```python
from build123d import *

# Parameters (mm, degrees)
SKETCH1_W           = 254
SKETCH1_H           = 31.75
SKETCH1_R           = 3.048
BOSS_EXTRUDE1_DEPTH = 2.54
CHAMFER1_SIZE       = 2.38
CHAMFER1_SIZE_2     = 4.122280922
SKETCH3_W           = 254
SKETCH3_H           = 12.7
BOSS_EXTRUDE2_DEPTH = 1.016
BOSS_EXTRUDE3_DEPTH = 1.016


with BuildPart() as part:
    # Sketch1 → Boss-Extrude1 (new body)
    with BuildSketch(Plane.XY):
        with Locations((127, 22.225)):
            Rectangle(SKETCH1_W, SKETCH1_H)
        with Locations((121.412, 12.7)):
            Circle(SKETCH1_R, mode=Mode.SUBTRACT)
        with Locations((248.412, 12.7)):
            Circle(SKETCH1_R, mode=Mode.SUBTRACT)
    extrude(amount=BOSS_EXTRUDE1_DEPTH)

    # Chamfer1
    # the kernel refuses this chamfer: 4.122280922, 2.38 mm, written as the material it takes off along each edge
    with BuildSketch(Plane(origin=(264.66469425, 6.35, 2.54), x_dir=(0, -0.05789386240267149, -0.9983227437537926), z_dir=(-1, 0, 0))) as chamfer1_piece_1:
        Polygon((CHAMFER1_SIZE * 0.998322743754, -CHAMFER1_SIZE * 0.0578938624027), (-CHAMFER1_SIZE_2 * 0.0578938624029, -CHAMFER1_SIZE_2 * 0.998322743757), (0, 0), align=None)
    extrude(amount=275.3293885, mode=Mode.SUBTRACT)

    # Sketch3 → Boss-Extrude2 (add)
    with BuildSketch(Plane(origin=(0, 0, 0), x_dir=(-1, 0, 0), z_dir=(0, 0, -1))):
        with Locations((-127, 31.75)):
            Rectangle(SKETCH3_W, SKETCH3_H)
    extrude(amount=BOSS_EXTRUDE2_DEPTH)

    # Sketch4 → Boss-Extrude3 (add)
    with BuildSketch(Plane(origin=(0, 0, 0), x_dir=(-1, 0, 0), z_dir=(0, 0, -1))):
        Polygon((0, 25.4), (0, 6.35), (-3.556, 6.35), (-14.224, 25.4), align=None)
    extrude(amount=BOSS_EXTRUDE3_DEPTH)


solid = part.part
```
The listing builds one solid part. Answer for the finished solid, in the listing's coordinates (mm). A direction names the side the tool comes from. Give positions to 0.01 mm unless a question says otherwise; leave off trailing zeros. Loops run counter-clockwise (first coordinate to the right, second up) from the corner with the lowest first, then second, coordinate; pieces in that order, holes last. Notation, with made-up numbers: M 82.25,26.5 L 137.25,26.5 A12 cw 137.25,49.5 Z; hole C -36,-39.75 d11. An arc over 180 degrees is marked long. One line per item, written item: value.
Q1. For faces 4 (the face through (125, 30, -1.016)), 5 (the face through (127, 16, 0)), determine the directions among +Z, -Z, +X, -X, +Y, -Y from which every point of the face is accessible in a straight line to the end or side of a thin tool.
Working result:
face 4: -Z, +X, -X, +Y, -Y
face 5: -Z, +X, -Y
Q2. A cutting plane is placed at A-A on x = 87. Determine the outline of the cut face in (y, z), then the cut area to 3 significant figures.
Working result:
outline: M 6.35,0 L 25.4,0 L 25.4,-1.02 L 38.1,-1.02 L 38.1,2.54 L 10.47,2.54 L 6.35,0.16 Z
area: 88.6 mm^2
Q3. A cutting plane is placed at B-B on y = 12.7. Determine the outline of the cut face in (x, z).
Working result:
outline: M 0,-1.02 L 7.11,-1.02 L 7.11,0 L 118.36,0 L 118.36,2.54 L 0,2.54 Z; M 124.46,0 L 245.36,0 L 245.36,2.54 L 124.46,2.54 Z; M 251.46,0 L 254,0 L 254,2.54 L 251.46,2.54 Z
Q4. Determine the mould class of faces 1 (the face through (121.015, 15.722, 1.252)), 2 (the face through (8.815, 15.742, -0.501)), 3 (the face through (125, 24, 2.54)) for opening direction X: +X half, -X half, draft (parallel to the pull), parting line (faces both ways), or undercut.
Working result:
face 1: undercut
face 2: +X half
face 3: draft
Q5. Find the intervals of material crossed by line 1 (X direction, y = 12.7, z = 1.8); line 2 (Y direction, x = 217.5, z = -0.4); line 3 (Z direction, x = 210.5, y = 23), in increasing order. Write a range as from..to.
Working result:
line 1: x = 0..118.36, 124.46..245.36, 251.46..254
line 2: y = 25.4..38.1
line 3: z = 0..2.54
Q6. A cutting plane is placed at C-C on z = 1.6. Determine the outline of the cut face in (x, y).
Working result:
outline: M 0,8.84 L 254,8.84 L 254,38.1 L 0,38.1 Z; hole C 121.41,12.7 d6.1; hole C 248.41,12.7 d6.1
Q7. Flat-ended cylindrical pins translate along their axes: P1, Ø1, axis at y = 17, z = 2, coming from the -X side; P2, Ø1, axis at x = 122, z = 1, coming from the -Y side; P3, Ø5, axis at x = 121.412, y = 12.7, coming from the -Z side; P4, Ø15, axis at x = 120, y = 12, coming from the -Z side. Find the tip coordinate at first contact, or state that the pin passes through.
Working result:
P1: stops at x = 0
P2: stops at y = 6.94
P3: passes through
P4: stops at z = 0
